Read the model definition and answer for the solid it produces. Units are mm, in the model's axes. Face numbers are marked on the shaded views. A direction names the side the tool comes from. Round coordinates to 2 decimals unless told otherwise and drop trailing zeros. Write each loop counter-clockwise with the first axis right and the second up, starting at its lowest first coordinate (ties: lowest second). Pieces come first, ordered by that corner, then holes. Notation, with made-up numbers: (-34, -35.5) -> (4, -35.5) arc R21 ccw to (4, -13.5) -> close; hole circle Ø8 at (51.5, 5). An arc over 180 degrees is marked (long way). Return JSON: item names as keys, results as strings. Group by question number.
(1) The mould has two halves that part along X. Classify the marked faces 4, 5, 6 and 7: released by +X, released by -X, zero draft, split by the parting line, or undercut.
(2) A cutting plane is placed at D-D on x = 53. Give the vertices of the cut face in (y, z).
(3) A cutting plane is placed at B-B on x = 204. Give the vertices of the cut face in (y, z).
(4) Given pin 1 (1.5 mm diameter, centred on y = 47, z = -124.5, fed in from +X); pin 2 (10 mm diameter, centred on x = 102.5, y = 116, fed in from -Z); pin 3 (10.5 mm diameter, centred on x = -5, y = -69.5, fed in from -Z); pin 4 (21.5 mm diameter, centred on x = -266.5, z = -32, fed in from +Y), each flat-ended and moving along its own axis, determine where each tip first touches the part or whether it passes through.
(5) A cutting plane is placed at A-A on z = -25.5. Give the vertices of the cut face in (x, y).
(6) For the marked faces 1, 2 and 3, determine the directions among +Z, -Z, +X, -X, +Y, -Y from which every point of the face is accessible in a straight line to the end or side of a thin tool.
(7) Straight lines are drawn through the part: line 1 (X direction, y = 200, z = -46.5); line 2 (Y direction, x = 171.5, z = -40.5); line 3 (Y direction, x = 278, z = -33.5). For each, find the intervals that lie inside material, in ascending order.
(8) A cutting plane is placed at C-C on y = 60.5. Give the vertices of the cut face in (x, z).
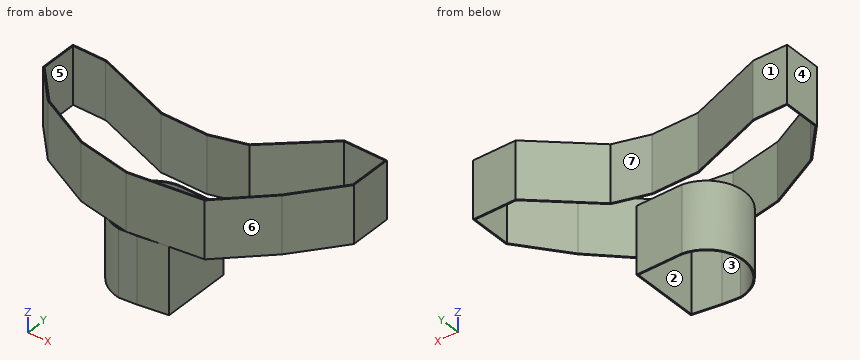
```python
from build123d import *

# Parameters (mm, degrees)
BOSS_EXTRUDE1_DEPTH = 120.65
BOSS_EXTRUDE2_DEPTH = 140.716


with BuildPart() as part:
    # Sketch1 → Boss-Extrude1 (new body)
    with BuildSketch(Plane.XY):
        Polygon((-291.084, 147.066), (-219.52806053, 147.066), (-57.22206053, 89.662), (39.256240725, 89.662), (110.476764153, 110.727225239), (226.088273147, 216.662), (316.23, 216.662), (316.23, 128.670079749), (241.68157023, 32.602515613), (150.279663639, -58.03130773), (-0.059802851, -78.008272613), (-110.526524053, -58.062892396), (-225.049772802, -2.07942928), (-291.084, 67.823990918), align=None)
        Polygon((111.76, 108.458), (39.624, 87.122), (-57.658, 87.122), (-219.964, 144.526), (-288.544, 144.526), (-288.544, 68.834), (-223.52, 0), (-109.728, -55.626), (0, -75.438), (149.098, -55.626), (239.776, 34.29), (313.69, 129.54), (313.69, 214.122), (227.076, 214.122), align=None, mode=Mode.SUBTRACT)
    extrude(amount=-BOSS_EXTRUDE1_DEPTH)

    # Sketch2 → Boss-Extrude2 (add)
    with BuildSketch(Plane(origin=(0, 0, -120.65), x_dir=(-1, 0, 0), z_dir=(0, 0, -1))):
        with BuildLine():
            Line((-81.788, 78.232), (14.098209979, 78.232))
            ThreePointArc((14.098209979, 78.232), (83.312, -0.762), (14.098209979, -79.756))
            Line((14.098209979, -79.756), (-21.914681881, -76.180251872))
            Line((-21.914681881, -76.180251872), (-81.788, -66.684923888))
            Line((-81.788, -66.684923888), (-81.788, 78.232))
        make_face()
        with BuildLine():
            Line((-79.248, 75.692), (-79.248, -64.516))
            Line((-79.248, -64.516), (-21.59, -73.66))
            Line((-21.59, -73.66), (14.224, -77.216))
            ThreePointArc((14.224, -77.216), (80.772, 0), (12.495590487, 75.692))
            Line((12.495590487, 75.692), (-79.248, 75.692))
        make_face(mode=Mode.SUBTRACT)
    extrude(amount=BOSS_EXTRUDE2_DEPTH)


solid = part.part
```
Checks:
{
 "1": {"face 4": "released by -X", "face 5": "undercut", "face 6": "released by +X", "face 7": "undercut"},
 "2": {"outline": "(-71.25, -261.37) -> (-68.68, -261.37) -> (-68.68, -120.65) -> (-68.4, -120.65) -> (-68.4, 0) -> (-70.96, 0) -> (-70.96, -120.65) -> (-71.25, -120.65) -> close; (75.69, -261.37) -> (78.23, -261.37) -> (78.23, -120.65) -> (75.69, -120.65) -> close; (91.08, -120.65) -> (93.73, -120.65) -> (93.73, 0) -> (91.08, 0) -> close"},
 "3": {"outline": "(-4.76, -120.65) -> (-1.19, -120.65) -> (-1.19, 0) -> (-4.76, 0) -> close; (192.98, -120.65) -> (196.42, -120.65) -> (196.42, 0) -> (192.98, 0) -> close"},
 "4": {"pin 1": "stops at x = 81.79", "pin 2": "passes through", "pin 3": "stops at z = -120.65", "pin 4": "stops at y = 147.07"},
 "5": {"outline": "(-291.08, 67.82) -> (-225.05, -2.08) -> (-110.53, -58.06) -> (-0.06, -78.01) -> (150.28, -58.03) -> (241.68, 32.6) -> (316.23, 128.67) -> (316.23, 216.66) -> (226.09, 216.66) -> (110.48, 110.73) -> (39.26, 89.66) -> (-57.22, 89.66) -> (-219.53, 147.07) -> (-291.08, 147.07) -> close; hole (-288.54, 68.83) -> (-223.52, 0) -> (-109.73, -55.63) -> (0, -75.44) -> (149.1, -55.63) -> (239.78, 34.29) -> (313.69, 129.54) -> (313.69, 214.12) -> (227.08, 214.12) -> (111.76, 108.46) -> (39.62, 87.12) -> (-57.66, 87.12) -> (-219.96, 144.53) -> (-288.54, 144.53) -> close"},
 "6": {"face 1": "+Z, -Z, -X, +Y", "face 2": "+Z, -Z", "face 3": "-Z"},
 "7": {"line 1": "x = 207.9 to 211.66, 313.69 to 316.23", "line 2": "y = -36.99 to -33.41, 163.2 to 166.64", "line 3": "y = 79.4 to 83.55, 214.12 to 216.66"},
 "8": {"outline": "(-284.17, -120.65) -> (-280.67, -120.65) -> (-280.67, 0) -> (-284.17, 0) -> close; (-54.58, -261.37) -> (-50.32, -261.37) -> (-50.32, -120.65) -> (-54.58, -120.65) -> close; (79.25, -261.37) -> (81.79, -261.37) -> (81.79, -120.65) -> (79.25, -120.65) -> close; (260.11, -120.65) -> (263.33, -120.65) -> (263.33, 0) -> (260.11, 0) -> close"}
}
